from build123d import *

# Parameters (mm, degrees)
F1_DEPTH = 25


with BuildPart() as f1:
    # F0 (on Top) → F1 (new body)
    with BuildSketch(Plane.XY):
        Polygon((-43.5267875595, 36.8303582072), (-43.5267875595, 11.1199722934), (-31.3423006786, 36.8303582072), align=None)
        with BuildLine():
            Line((-43.5267875595, 36.8303582072), (-31.3423006786, 36.8303582072))
            Line((-31.3423006786, 36.8303582072), (-16.9682625481, 67.1608982694))
            ThreePointArc((-16.9682625481, 67.1608982694), (-35.9487677178, 56.9878438592), (-43.5267875595, 36.8303582072))
        make_face()
        with BuildLine():
            ThreePointArc((8.1727226195, 58.9890034381), (-6.6535791829, 52.0475969983), (-12.689968176, 36.8303582072))
            Line((-12.689968176, 36.8303582072), (9.508928284, 36.8303582072))
            Line((9.508928284, 36.8303582072), (9.508928284, 14.6314617472))
            ThreePointArc((9.508928284, 14.6314617472), (25.2059185058, 21.1333679855), (31.7078247441, 36.8303582072))
            ThreePointArc((31.7078247441, 36.8303582072), (24.7261670751, 52.9928656742), (8.1727226195, 58.9890034381))
        make_face()
        with BuildLine():
            Line((9.508928284, 36.8303582072), (-12.689968176, 36.8303582072))
            ThreePointArc((-12.689968176, 36.8303582072), (-6.1880619377, 21.1333679855), (9.508928284, 14.6314617472))
            Line((9.508928284, 14.6314617472), (9.508928284, 36.8303582072))
        make_face()
        with BuildLine():
            Line((-31.3423006786, 36.8303582072), (-43.5267875595, 11.1199722934))
            Line((-43.5267875595, 11.1199722934), (9.508928284, 11.1199722934))
            Line((9.508928284, 11.1199722934), (9.508928284, 14.6314617472))
            ThreePointArc((9.508928284, 14.6314617472), (-6.1880619377, 21.1333679855), (-12.689968176, 36.8303582072))
            Line((-12.689968176, 36.8303582072), (-31.3423006786, 36.8303582072))
        make_face()
        with BuildLine():
            Line((-16.9682625481, 67.1608982694), (-31.3423006786, 36.8303582072))
            Line((-31.3423006786, 36.8303582072), (-12.689968176, 36.8303582072))
            ThreePointArc((-12.689968176, 36.8303582072), (-6.6535791829, 52.0475969983), (8.1727226195, 58.9890034381))
            ThreePointArc((8.1727226195, 58.9890034381), (-3.4697191171, 65.9301164017), (-16.9682625481, 67.1608982694))
        make_face()
    extrude(amount=F1_DEPTH)


solid = f1.part
Part model, mm, in its own coordinate system. A direction names the side the tool comes from. Coordinates: 2 decimals unless noted, no trailing zeros. Loops run counter-clockwise (first coordinate to the right, second up) from the corner with the lowest first, then second, coordinate; pieces in that order, holes last. Notation, with made-up numbers: (-3, 36.25) -> (1, 36.25) arc R9 ccw to (1, 43.25) -> close; hole circle Ø1 at (10, -37). An arc over 180 degrees is marked (long way). Use a Markdown table: item, result. Add a question column.
Item 1: Band-saw the part on A-A on z = 14.25. Write the cut outline in (x, y), plus the area to 3 significant figures.
Item 2: Band-saw the part on C-C on x = -37. Write the cut outline in (y, z), plus the area to 4 significant figures.
Item 3: Band-saw the part on B-B on y = 25.5. Write the cut outline in (x, z), plus the area to 3 significant figures.
Item 4: Which spindle directions (+Z, -Z, +X, -X, +Y, -Y) get a long thin tool onto all of the face, cutting with end or side? Do faces 1 (the flat face through (9.509, 13, 12)), 2 (the flat face through (-17, 11.12, 12)). Say none if no direction does.
Item 5: Flat gauge pin, fed straight in: P1, Ø1, axis at y = 45, z = 18, coming from the -X side. Where does the tip first touch, or does it go through?
Item 6: Probe probe 1 along X at (y, z) = (14.5, 14); probe 2 along Y at (x, z) = (-12.5, 19); probe 3 along Y at (x, z) = (8, 2.75). List the from-to ranges inside material, lowest first.
Geometry says:
| question | item | result |
|---|---|---|
| 1 | outline | (-43.53, 11.12) -> (9.51, 11.12) -> (9.51, 14.63) arc R22.2 ccw (long way) to (8.17, 58.99) arc R30.6 ccw to (-43.53, 36.83) -> close |
| 1 | area | 3,490 mm² |
| 2 | outline | (11.12, 0) -> (55.72, 0) -> (55.72, 25) -> (11.12, 25) -> close |
| 2 | area | 1,115 mm² |
| 3 | outline | (-43.53, 0) -> (28.6, 0) -> (28.6, 25) -> (-43.53, 25) -> close |
| 3 | area | 1,800 mm² |
| 4 | face 1 | +Z, -Z, +X, -Y |
| 4 | face 2 | +Z, -Z, +X, -X, -Y |
| 5 | P1 | x = -42.55 |
| 6 | probe 1 | -43.53 to 9.51 |
| 6 | probe 2 | 11.12 to 67.43 |
| 6 | probe 3 | 11.12 to 59.15 |
